```python
from build123d import *

# Parameters (mm, degrees)
EXTRUDE_1_DEPTH     = 300
SKETCH_2_R          = 5
CUT_EXTRUDE_1_DEPTH = 33
CHAMFER_1_SIZE      = 1


with BuildPart() as part:
    # Эскиз1 → Вытянуть-Тонкостенный1 (new body)
    with BuildSketch(Plane(origin=(0, 0, 0), x_dir=(1, 0, 0), z_dir=(0, 1, 0))):
        Polygon((0, 32), (0, 0), (32, 0), (32, 3), (3, 3), (3, 32), align=None)
    extrude(amount=EXTRUDE_1_DEPTH)

    # Эскиз2 → Вырез-Вытянуть1 (cut, through all)
    with BuildSketch(Plane.XY):
        with Locations((22, 10)):
            Circle(SKETCH_2_R)
        with Locations((22, 150)):
            Circle(SKETCH_2_R)
        with Locations((22, 290)):
            Circle(SKETCH_2_R)
    extrude(amount=-CUT_EXTRUDE_1_DEPTH, mode=Mode.SUBTRACT)

    # Фаска1
    chamfer_1_edges = [part.edges().sort_by_distance(p)[0] for p in [
        (17, 10, -3),
        (17, 150, -3),
        (17, 290, -3),
    ]]
    chamfer(chamfer_1_edges, length=CHAMFER_1_SIZE)


solid = part.part
```
Geometry check sheet. Reference: the model listing, model coordinates, mm. A direction names the side the tool comes from. Round coordinates to 2 decimals unless told otherwise and drop trailing zeros. Order: outer loops, then holes, each group sorted by start corner. A loop starts at its lowest first (then second) coordinate and runs counter-clockwise, first axis right, second up. Notation, with made-up numbers: M 56.25,63 L 113.25,63 A19 ccw 113.25,79 Z; hole C -32,81 d1. An arc over 180 degrees is marked long. Write item = value, one per line.
Q1. Section check B-B (x = 22). Enter the section's corners in (y, z).
Answer block:
outline = M 0,-3 L 4,-3 L 5,-2 L 5,0 L 0,0 Z; M 15,-2 L 16,-3 L 144,-3 L 145,-2 L 145,0 L 15,0 Z; M 155,-2 L 156,-3 L 284,-3 L 285,-2 L 285,0 L 155,0 Z; M 295,-2 L 296,-3 L 300,-3 L 300,0 L 295,0 Z
Q2. Section check A-A (y = 290). Enter the section's corners in (x, z).
Answer block:
outline = M 0,-32 L 3,-32 L 3,-3 L 16,-3 L 17,-2 L 17,0 L 0,0 Z; M 27,-2 L 28,-3 L 32,-3 L 32,0 L 27,0 Z
Q3. Depth check by flat-ended pin: pin 1 Ø2 at (y, z) = (95.5, -9.5) entering from -X; pin 2 Ø6 at (x, y) = (22, 290) entering from -Z; pin 3 Ø1.5 at (y, z) = (214, -11.5) entering from +X; pin 4 Ø4 at (x, y) = (24.5, 232) entering from -Z. Enter the tip coordinate at first touch or a pass-through.
Answer block:
pin_1 = 0
pin_2 = through
pin_3 = 3
pin_4 = -3
Q4. Set-up check for faces 4 (the cylindrical face through (21.349, 294.957, -0.986)), 5 (the flat face through (3, 148, -17)): record each of +Z, -Z, +X, -X, +Y, -Y from which the full face is reachable in a straight line by a thin tool's end or side.
Answer block:
face_4 = +Z, -Z
face_5 = -Z, +X, +Y, -Y
Q5. Section check D-D (z = -14.5). Enter the section's corners in (x, y).
Answer block:
outline = M 0,0 L 3,0 L 3,300 L 0,300 Z
Q6. Scan lines: line 1 (Y direction, x = 22, z = -1); line 2 (X direction, y = 290, z = -0.7); line 3 (Z direction, x = 12, y = 232). Record each from-to range of solid material in increasing order.
Answer block:
line_1 = 0 to 5, 15 to 145, 155 to 285, 295 to 300
line_2 = 0 to 17, 27 to 32
line_3 = -3 to 0
Q7. Section check C-C (y = 169.5). Enter the section's corners in (x, z).
Answer block:
outline = M 0,-32 L 3,-32 L 3,-3 L 32,-3 L 32,0 L 0,0 Z
Q8. Release check for a two-part mould opening along Y. For faces 1 (the flat face through (2, 300, -10)), 2 (the cylindrical face through (20.92, 145.12, -0.99)), 3 (the flat face through (2, 0, -10)) record: released by +Y, released by -Y, zero draft, split by the parting line, or undercut.
Answer block:
face_1 = released by +Y
face_2 = undercut
face_3 = released by -Y
